```python
from build123d import *
from OCP.BRepFilletAPI import BRepFilletAPI_MakeChamfer

# Parameters (mm, degrees)
SKETCH5_R           = 1.7
BOSS_EXTRUDE1_DEPTH = 2
SKETCH9_R           = 1.7
BOSS_EXTRUDE3_DEPTH = 3
BOSS_EXTRUDE4_DEPTH = 3.6
BOSS_EXTRUDE5_DEPTH = 7.8
TOP_ANGLE_1_DEPTH   = 25
TOP_ANGLE_2_DEPTH   = 25
CHAMFER1_SIZE       = 3
CHAMFER1_SIZE_2     = 3.575260778
CHAMFER2_SIZE       = 1.8
CHAMFER2_SIZE2      = 2.145156467
SKETCH19_R          = 1.7
CUT_EXTRUDE1_DEPTH  = 3.75
M3_HEAD_HOLES_DEPTH = 3
CHAMFER3_SIZE       = 0.5


# Some blends are built 0.0001 mm under size
with BuildPart() as part:
    # Sketch5 → Boss-Extrude1 (new body)
    with BuildSketch(Plane.XY):
        Polygon((16.5, 44.802943725), (16.5, 45.24192642), (16.5, 61.363961031), (17, 61.863961031), (19.636038969, 64.5), (23.363961031, 64.5), (26, 61.863961031), (26, 58.136038969), (23.363961031, 55.5), (21.5, 53.636038969), (21.5, 43.64192642), (23.363961031, 41.777965389), (23.363961031, 37.5), (26, 34.863961031), (26, 31.136038969), (23.363961031, 28.5), (18.5, 23.636038969), (18.5, 13.64192642), (20.338982694, 11.802943725), (23.363961031, 8.777965389), (23.363961031, 4.5), (26, 1.863961031), (26, -1.863961031), (23.363961031, -4.5), (19.636038969, -4.5), (17, -1.863961031), (17, 0), (-17, 0), (-17, -1.863961031), (-19.636038969, -4.5), (-23.363961031, -4.5), (-26, -1.863961031), (-26, 1.863961031), (-23.363961031, 4.5), (-23.363961031, 8.777965389), (-20.338982694, 11.802943725), (-18.5, 13.64192642), (-18.5, 23.636038969), (-23.363961031, 28.5), (-26, 31.136038969), (-26, 34.863961031), (-23.363961031, 37.5), (-23.363961031, 41.777965389), (-21.5, 43.64192642), (-21.5, 53.636038969), (-23.363961031, 55.5), (-26, 58.136038969), (-26, 61.863961031), (-23.363961031, 64.5), (-19.636038969, 64.5), (-17, 61.863961031), (-16.5, 61.363961031), (-16.5, 60), (-16.5, 44.802943725), (-16.061017306, 44.802943725), (-14, 44.802943725), (-14, 42.74192642), (-13.036038969, 41.777965389), (-12, 40.74192642), (-12, 29.029437252), (-4.970562748, 22), (4.970562748, 22), (12, 29.029437252), (12, 40.74192642), (13.036038969, 41.777965389), (14, 42.74192642), (14, 44.802943725), (16.061017306, 44.802943725), align=None)
        with Locations((-18.2, 6.638982694)):
            Circle(SKETCH5_R, mode=Mode.SUBTRACT)
        with Locations((-18.2, 39.638982694)):
            Circle(SKETCH5_R, mode=Mode.SUBTRACT)
        with Locations(Location((18.2, 39.638982694, 0), (0, 0, 180))):
            Circle(SKETCH5_R, mode=Mode.SUBTRACT)
        with Locations(Location((18.2, 6.638982694, 0), (0, 0, 180))):
            Circle(SKETCH5_R, mode=Mode.SUBTRACT)
        Polygon((5.798989873, 2), (-5.798989873, 2), (-12, 8.201010127), (-12, 26.201010127), (-5.798989873, 20), (5.798989873, 20), (12, 26.201010127), (12, 8.201010127), align=None, mode=Mode.SUBTRACT)
    extrude(amount=BOSS_EXTRUDE1_DEPTH)

    # Sketch9 → Boss-Extrude3 (add)
    with BuildSketch(Plane.XY.offset(2)):
        Polygon((-19.636038969, -4.5), (-17, -1.863961031), (-17, 1.475021664), (-16.061017306, 1.475021664), (-13.036038969, 4.5), (-13.036038969, 8.777965389), (-16.061017306, 11.802943725), (-16.5, 11.802943725), (-16.5, 34.363961031), (-16.5, 34.475021664), (-16.061017306, 34.475021664), (-14, 36.536038969), (-14, 28.201010127), (-12, 26.201010127), (-5.798989873, 20), (5.798989873, 20), (12, 26.201010127), (14, 28.201010127), (14, 36.536038969), (16.061017306, 34.475021664), (16.5, 34.475021664), (16.5, 34.363961031), (16.5, 11.802943725), (16.061017306, 11.802943725), (13.036038969, 8.777965389), (13.036038969, 4.5), (16.061017306, 1.475021664), (17, 1.475021664), (17, -1.863961031), (19.636038969, -4.5), (23.363961031, -4.5), (26, -1.863961031), (26, 1.863961031), (23.363961031, 4.5), (23.363961031, 8.777965389), (20.338982694, 11.802943725), (18.5, 13.64192642), (18.5, 23.636038969), (23.363961031, 28.5), (26, 31.136038969), (26, 34.863961031), (23.363961031, 37.5), (23.363961031, 41.777965389), (21.5, 43.64192642), (21.5, 53.636038969), (23.363961031, 55.5), (26, 58.136038969), (26, 61.863961031), (23.363961031, 64.5), (19.636038969, 64.5), (17, 61.863961031), (16.5, 61.363961031), (16.5, 45.24192642), (16.5, 44.802943725), (16.061017306, 44.802943725), (14, 44.802943725), (14, 42.74192642), (13.036038969, 41.777965389), (12, 40.74192642), (12, 29.029437252), (4.970562748, 22), (-4.970562748, 22), (-12, 29.029437252), (-12, 40.74192642), (-13.036038969, 41.777965389), (-14, 42.74192642), (-14, 44.802943725), (-16.061017306, 44.802943725), (-16.5, 44.802943725), (-16.5, 60), (-16.5, 61.363961031), (-17, 61.863961031), (-19.636038969, 64.5), (-23.363961031, 64.5), (-26, 61.863961031), (-26, 58.136038969), (-23.363961031, 55.5), (-21.5, 53.636038969), (-21.5, 43.64192642), (-23.363961031, 41.777965389), (-23.363961031, 37.5), (-26, 34.863961031), (-26, 31.136038969), (-23.363961031, 28.5), (-18.5, 23.636038969), (-18.5, 13.64192642), (-20.338982694, 11.802943725), (-23.363961031, 8.777965389), (-23.363961031, 4.5), (-26, 1.863961031), (-26, -1.863961031), (-23.363961031, -4.5), align=None)
        with Locations((-21.5, 33)):
            Circle(SKETCH9_R, mode=Mode.SUBTRACT)
        with Locations((-18.2, 39.638982694)):
            Circle(SKETCH9_R, mode=Mode.SUBTRACT)
        with Locations((-21.5, 0)):
            Circle(SKETCH9_R, mode=Mode.SUBTRACT)
        with Locations((-18.2, 6.638982694)):
            Circle(SKETCH9_R, mode=Mode.SUBTRACT)
        with Locations(Location((18.2, 6.638982694, 0), (0, 0, 180))):
            Circle(SKETCH9_R, mode=Mode.SUBTRACT)
        with Locations(Location((21.5, 0, 0), (0, 0, 180))):
            Circle(SKETCH9_R, mode=Mode.SUBTRACT)
        with Locations(Location((18.2, 39.638982694, 0), (0, 0, 180))):
            Circle(SKETCH9_R, mode=Mode.SUBTRACT)
        with Locations(Location((21.5, 33, 0), (0, 0, 180))):
            Circle(SKETCH9_R, mode=Mode.SUBTRACT)
    extrude(amount=BOSS_EXTRUDE3_DEPTH)

    # Sketch10 → Boss-Extrude4 (add)
    with BuildSketch(Plane.XY.offset(5)):
        Polygon((17, 58.136038969), (16.5, 58.636038969), (16.5, 61.363961031), (17, 61.863961031), (19.636038969, 64.5), (23.363961031, 64.5), (26, 61.863961031), (26, 58.136038969), (23.363961031, 55.5), (21.5, 53.636038969), (19.636038969, 55.5), align=None)
        Polygon((-17, 61.863961031), (-19.636038969, 64.5), (-23.363961031, 64.5), (-26, 61.863961031), (-26, 58.136038969), (-23.363961031, 55.5), (-21.5, 53.636038969), (-19.636038969, 55.5), (-17, 58.136038969), (-16.5, 58.636038969), (-16.5, 61.363961031), align=None)
    extrude(amount=BOSS_EXTRUDE4_DEPTH)

    # Sketch20 → Boss-Extrude5 (add)
    with BuildSketch(Plane.XY.offset(8.6)):
        Polygon((-17, 58.136038969), (-17, 61.863961031), (-19.636038969, 64.5), (-23.363961031, 64.5), (-26, 61.863961031), (-26, 58.136038969), (-23.363961031, 55.5), (-19.636038969, 55.5), align=None)
        Polygon((17, 61.863961031), (19.636038969, 64.5), (23.363961031, 64.5), (26, 61.863961031), (26, 58.136038969), (23.363961031, 55.5), (19.636038969, 55.5), (17, 58.136038969), align=None)
    extrude(amount=BOSS_EXTRUDE5_DEPTH)

    # Sketch15 → Top Angle 1 (cut, symmetric)
    with BuildSketch(Plane(origin=(19.25, 19.25, 0), x_dir=(0, 0, -1), z_dir=(0.7071067811865485, 0.7071067811865467, 0))):
        Polygon((0, 53.129202667), (-15.320888862, 65.98495486), (-8.893012766, 73.645399292), (6.427876097, 60.789647098), align=None)
    extrude(amount=TOP_ANGLE_1_DEPTH, both=True, mode=Mode.SUBTRACT)

    # Sketch16 → Top Angle 2 (cut, symmetric)
    with BuildSketch(Plane(origin=(-19.25, 19.25, 0), x_dir=(0.7071067811865475, 0.7071067811865477, 0), z_dir=(-0.7071067811865477, 0.7071067811865475, 0))):
        Polygon((53.129202667, 0), (65.98495486, -15.320888862), (73.645399292, -8.893012766), (60.789647098, 6.427876097), align=None)
    extrude(amount=TOP_ANGLE_2_DEPTH, both=True, mode=Mode.SUBTRACT)

    # Chamfer1
    # the kernel refuses this chamfer: 3.575260778, 3 mm, written as the material it adds along each edge
    with BuildSketch(Plane(origin=(-28.015917535, 47.120121434, 5), x_dir=(0.7066633444206492, -0.7066633444206532, -0.03540953691366292), z_dir=(0.7071067811865496, 0.7071067811865456, 0))) as chamfer1_piece_1_section:
        Polygon((CHAMFER1_SIZE * 0.999372885712, -CHAMFER1_SIZE * 0.0354095369137), (-CHAMFER1_SIZE_2 * 0.0354095369115, -CHAMFER1_SIZE_2 * 0.999372885651), (0, 0), align=None)
    chamfer1_piece_1 = extrude(amount=25.500865711, mode=Mode.PRIVATE)
    chamfer1_piece_1 = split(chamfer1_piece_1, bisect_by=Plane(origin=(-21.5, 51.974230038, 5.812222145), z_dir=(1, 0, 0)), keep=Keep.TOP, mode=Mode.PRIVATE)
    chamfer1_piece_1 = split(chamfer1_piece_1, bisect_by=Plane(origin=(-20.392127379, 52.528166349, 5.812222145), z_dir=(-0.7071067811865449, -0.7071067811865502, 0)), keep=Keep.TOP, mode=Mode.PRIVATE)
    add(chamfer1_piece_1)
    with BuildSketch(Plane(origin=(-21.5, 53.636038969, 5), x_dir=(0.7066633444206492, -0.7066633444206532, -0.03540953691366292), z_dir=(0.7071067811865496, 0.7071067811865456, 0))) as chamfer1_piece_2_section:
        Polygon((CHAMFER1_SIZE * 0.999372885712, -CHAMFER1_SIZE * 0.0354095369137), (-CHAMFER1_SIZE_2 * 0.0354095369115, -CHAMFER1_SIZE_2 * 0.999372885651), (0, 0), align=None)
    chamfer1_piece_2 = extrude(amount=16.285966762, mode=Mode.PRIVATE)
    chamfer1_piece_2 = split(chamfer1_piece_2, bisect_by=Plane(origin=(-21.5, 55.195385709, 6.244922793), z_dir=(1, 0, 0)), keep=Keep.TOP, mode=Mode.PRIVATE)
    chamfer1_piece_2 = split(chamfer1_piece_2, bisect_by=Plane(origin=(-16.5, 55.195385709, 6.244922793), z_dir=(-1, 0, 0)), keep=Keep.TOP, mode=Mode.PRIVATE)
    add(chamfer1_piece_2)
    with BuildSketch(Plane(origin=(9.984082465, 65.151956505, 5), x_dir=(0.017634763768199533, 0.01763476376819963, 0.9996889667359942), z_dir=(0.7071067811865496, -0.7071067811865456, 0))) as chamfer1_piece_3_section:
        Polygon((CHAMFER1_SIZE_2 * 0.999688966675, CHAMFER1_SIZE_2 * 0.0249393220887), (-CHAMFER1_SIZE * 0.0249393220902, CHAMFER1_SIZE * 0.999688966736), (0, 0), align=None)
    chamfer1_piece_3 = extrude(amount=16.285966762, mode=Mode.PRIVATE)
    chamfer1_piece_3 = split(chamfer1_piece_3, bisect_by=Plane(origin=(16.5, 55.195385709, 6.244922793), z_dir=(1, 0, 0)), keep=Keep.TOP, mode=Mode.PRIVATE)
    chamfer1_piece_3 = split(chamfer1_piece_3, bisect_by=Plane(origin=(21.5, 55.195385709, 6.244922793), z_dir=(-1, 0, 0)), keep=Keep.TOP, mode=Mode.PRIVATE)
    add(chamfer1_piece_3)
    with BuildSketch(Plane(origin=(9.984082465, 65.151956505, 5), x_dir=(0.017634763768199533, 0.01763476376819963, 0.9996889667359942), z_dir=(0.7071067811865496, -0.7071067811865456, 0))) as chamfer1_piece_4_section:
        Polygon((CHAMFER1_SIZE_2 * 0.999688966675, CHAMFER1_SIZE_2 * 0.0249393220887), (-CHAMFER1_SIZE * 0.0249393220902, CHAMFER1_SIZE * 0.999688966736), (0, 0), align=None)
    chamfer1_piece_4 = extrude(amount=25.500865711, mode=Mode.PRIVATE)
    chamfer1_piece_4 = split(chamfer1_piece_4, bisect_by=Plane(origin=(20.392127379, 52.528166349, 5.812222145), z_dir=(0.707106781186548, -0.707106781186547, 0)), keep=Keep.TOP, mode=Mode.PRIVATE)
    chamfer1_piece_4 = split(chamfer1_piece_4, bisect_by=Plane(origin=(21.5, 51.974230038, 5.812222145), z_dir=(-1, 0, 0)), keep=Keep.TOP, mode=Mode.PRIVATE)
    add(chamfer1_piece_4)

    # Chamfer2: one chamfer whose edges measure the first distance from different faces: ONE call of the kernel's chamfer builder (chamfer() names one face for all edges)
    chamfer2_edges_1 = [part.edges().sort_by_distance(p)[0] for p in [
        (21.5, 55.5, 8.6),
    ]]
    chamfer2_side_1 = [part.faces().sort_by_distance(p)[0] for p in [
        (21.5, 54.878679656, 8.6),
    ]]
    chamfer2_edges_2 = [part.edges().sort_by_distance(p)[0] for p in [
        (-21.5, 55.5, 8.6),
    ]]
    chamfer2_side_2 = [part.faces().sort_by_distance(p)[0] for p in [
        (-21.5, 54.878679656, 8.6),
    ]]
    chamfer2 = BRepFilletAPI_MakeChamfer(part.part.solid().wrapped)
    for e in chamfer2_edges_1:
        chamfer2.Add(CHAMFER2_SIZE, CHAMFER2_SIZE2, e.wrapped, chamfer2_side_1[0].wrapped)  # the first distance lies on this face
    for e in chamfer2_edges_2:
        chamfer2.Add(CHAMFER2_SIZE, CHAMFER2_SIZE2, e.wrapped, chamfer2_side_2[0].wrapped)  # the first distance lies on this face
    add(Compound.cast(chamfer2.Shape()), mode=Mode.REPLACE)

    # Sketch19 → Cut-Extrude1 (cut)
    with BuildSketch(Plane.XY.offset(16.4)):
        with Locations((-21.5, 60)):
            Circle(SKETCH19_R)
        with Locations((21.5, 60)):
            Circle(SKETCH19_R)
    extrude(amount=-CUT_EXTRUDE1_DEPTH, mode=Mode.SUBTRACT)

    # Sketch18 → M3 Head Holes (cut)
    with BuildSketch(Plane(origin=(0, 0, 0), x_dir=(-1, 0, 0), z_dir=(0, 0, -1))):
        Polygon((16.496816706, 42.588982694), (19.903183294, 42.588982694), (21.606366588, 39.638982694), (19.903183294, 36.688982694), (16.496816706, 36.688982694), (14.793633412, 39.638982694), align=None)
        Polygon((19.903183294, 9.588982694), (21.606366588, 6.638982694), (19.903183294, 3.688982694), (16.496816706, 3.688982694), (14.793633412, 6.638982694), (16.496816706, 9.588982694), align=None)
        Polygon((-21.606366588, 6.638982694), (-19.903183294, 3.688982694), (-16.496816706, 3.688982694), (-14.793633412, 6.638982694), (-16.496816706, 9.588982694), (-19.903183294, 9.588982694), align=None)
        Polygon((-14.793633412, 39.638982694), (-16.496816706, 42.588982694), (-19.903183294, 42.588982694), (-21.606366588, 39.638982694), (-19.903183294, 36.688982694), (-16.496816706, 36.688982694), align=None)
    extrude(amount=-M3_HEAD_HOLES_DEPTH, mode=Mode.SUBTRACT)

    # Chamfer3
    chamfer3_edges = [part.edges().sort_by_distance(p)[0] for p in [
        (17, 60, 8.6),
        (-17, 60, 8.6),
    ]]
    chamfer(chamfer3_edges, length=CHAMFER3_SIZE - 0.0001)  # a hair under: the kernel refuses the full size


solid = part.part
```
Here's how the part is built. I have some questions about the finished solid (model axes, mm). A direction names the side the tool comes from. Give positions to 0.01 mm unless a question says otherwise; leave off trailing zeros. Write each loop counter-clockwise with the first axis right and the second up, starting at its lowest first coordinate (ties: lowest second). Pieces come first, ordered by that corner, then holes.
(1) Imagine slicing it at A-A, the plane y = 46. Write out the boundary of the cut face in (x, z), and give its area (3 significant figures).
Output values:
outline: (-21.5, 0) - (-16.5, 0) - (-16.5, 5) - (-21.5, 5) - close; (16.5, 0) - (21.5, 0) - (21.5, 5) - (16.5, 5) - close
area: 50.0 mm2
(2) If I drill on L1, parallel to X at y = 25, z = 4.75; L2, parallel to X at y = 58.5, z = 9.25; L3, parallel to Y at x = 18, z = 4.25, over which ranges is the centre line in solid material (lowest first)?
Output values:
L1: x = -19.86 to -16.5, -10.8 to -7.97, 7.97 to 10.8, 16.5 to 19.86
L2: x = -26 to -17, 17 to 26
L3: y = -2.86 to 4.95, 8.33 to 37.95, 41.33 to 62.18
(3) Imagine slicing it at B-B, the plane z = 14.5. Write out the boundary of the cut face in (x, y).
Output values:
outline: (-26, 58.14) - (-23.36, 55.5) - (-19.64, 55.5) - (-17, 58.14) - (-17, 61.86) - (-19.64, 64.5) - (-23.36, 64.5) - (-26, 61.86) - close; (17, 58.14) - (19.64, 55.5) - (23.36, 55.5) - (26, 58.14) - (26, 61.86) - (23.36, 64.5) - (19.64, 64.5) - (17, 61.86) - close; hole circle Ø3.4 at (-21.5, 60); hole circle Ø3.4 at (21.5, 60)
(4) On a 3-axis mill with a long thin cutter (end or side, diameter ignored), from which of +Z, -Z, +X, -X, +Y, -Y can I reach the whole of each face in a straight line? I mean faces 5 (the face through (15.66, 38.14, 1.48)), 6 (the face through (20.7, 34.5, 3.5)), 7 (the face through (-24.664, 3.2, 2.465)), 8 (the face through (-12, 17, 1)). Say none if no direction works.
Output values:
face 5: -Z
face 6: +Z
face 7: +Z, -Z, -X
face 8: +Z, -Z
(5) Will these pins go through, and if not, where does the flat tip stop? pin 1 (1 mm diameter, centred on x = -21.5, y = -1, fed in from +Z); pin 2 (3.5 mm diameter, centred on x = 21, y = 60.5, fed in from +Z); pin 3 (6 mm diameter, centred on x = -0.5, y = 18.5, fed in from +Z); pin 4 (2.5 mm diameter, centred on x = -19, z = 1.5, fed in from +Y).
Output values:
pin 1: stops at z = 2
pin 2: stops at z = 16.4
pin 3: stops at z = 5
pin 4: stops at y = 59.86
(6) Imagine slicing it at C-C, the plane x = -7. Write out the boundary of the cut face in (y, z), and give its area (3 significant figures).
Output values:
outline: (0, 0) - (3.2, 0) - (3.2, 2) - (0, 2) - close; (21.2, 0) - (24.03, 0) - (24.03, 5) - (21.2, 5) - close
area: 20.5 mm2
(7) Imagine slicing it at D-D, the plane y = 33. Write out the boundary of the cut face in (x, z), and give its area (3 significant figures).
Output values:
outline: (-26, 0) - (-12, 0) - (-12, 5) - (-14, 5) - (-14, 2) - (-16.5, 2) - (-16.5, 5) - (-19.8, 5) - (-19.8, 2) - (-23.2, 2) - (-23.2, 5) - (-26, 5) - close; (12, 0) - (26, 0) - (26, 5) - (23.2, 5) - (23.2, 2) - (19.8, 2) - (19.8, 5) - (16.5, 5) - (16.5, 2) - (14, 2) - (14, 5) - (12, 5) - close
area: 105 mm2
(8) Thinking about a two-plate mould opening in Y: for faces 1 (the face through (-19.035, 53.95, 6.763)), 2 (the face through (-19.9, 39.7, 4)), 3 (the face through (-21, 64.5, 13)), 4 (the face through (26, 33, 2)), which applies, pulls with the +Y half, pulls with the -Y half, needs draft (parallel to the pull), parting line crosses it, or undercut?
Output values:
face 1: pulls with the -Y half
face 2: undercut
face 3: pulls with the +Y half
face 4: needs draft
